from build123d import *

# Parameters (mm, degrees)
SKETCH1_W           = 36
SKETCH1_H           = 42
SKETCH1_R           = 1.55
BOSS_EXTRUDE1_DEPTH = 2
SKETCH5_W           = 42
SKETCH5_H           = 9.1
BOSS_EXTRUDE2_DEPTH = 7.4
SKETCH6_W           = 10
SKETCH6_H           = 9.1
BOSS_EXTRUDE3_DEPTH = 2
SKETCH2_R           = 3
CUT_EXTRUDE1_DEPTH  = 6
SKETCH4_W           = 16
SKETCH4_H           = 1.45
BOSS_EXTRUDE4_DEPTH = 0.4
FILLET2_R           = 3
FILLET3_R           = 0.5
SKETCH7_W           = 29
SKETCH7_H           = 20
BOSS_EXTRUDE5_DEPTH = 6
SKETCH8_W           = 20
SKETCH8_H           = 20
SKETCH8_R           = 8
SKETCH8_R_2         = 1.05
BOSS_EXTRUDE6_DEPTH = 3
FILLET4_R           = 2
SKETCH10_W          = 24
SKETCH10_H          = 19
SKETCH10_R          = 2.6
BOSS_EXTRUDE7_DEPTH = 3
SKETCH14_W          = 26
SKETCH14_H          = 25
BOSS_EXTRUDE8_DEPTH = 10.5
CUT_EXTRUDE3_REACH  = 60.08
SKETCH9_R           = 3.25
CUT_EXTRUDE2_DEPTH  = 13
FILLET6_R           = 1
FILLET7_R           = 1
FILLET8_R           = 4
FILLET9_R           = 1
FILLET10_R          = 1


with BuildPart() as part:
    # Sketch1 → Boss-Extrude1 (new body)
    with BuildSketch(Plane(origin=(0, 0, 0), x_dir=(0, 1, 0), z_dir=(0, 0, 1))):
        with Locations((5, 0)):
            Rectangle(SKETCH1_W, SKETCH1_H)
        with Locations(Location((-10, -10, 0), (0, 0, 270))):
            Circle(SKETCH1_R, mode=Mode.SUBTRACT)
        with Locations(Location((10, -10, 0), (0, 0, 270))):
            Circle(SKETCH1_R, mode=Mode.SUBTRACT)
        with Locations(Location((10, 10, 0), (0, 0, 270))):
            Circle(SKETCH1_R, mode=Mode.SUBTRACT)
        with Locations(Location((-10, 10, 0), (0, 0, 270))):
            Circle(SKETCH1_R, mode=Mode.SUBTRACT)
    extrude(amount=BOSS_EXTRUDE1_DEPTH)

    # Sketch5 → Boss-Extrude2 (add)
    with BuildSketch(Plane.XY):
        with Locations((0, 18.45)):
            Rectangle(SKETCH5_W, SKETCH5_H)
    extrude(amount=-BOSS_EXTRUDE2_DEPTH)

    # Sketch6 → Boss-Extrude3 (add)
    with BuildSketch(Plane(origin=(0, 0, -7.4), x_dir=(1, 0, 0), z_dir=(0, 0, -1))):
        with Locations((0, -18.45)):
            Rectangle(SKETCH6_W, SKETCH6_H)
    extrude(amount=BOSS_EXTRUDE3_DEPTH)

    # Sketch2 → Cut-Extrude1 (cut)
    with BuildSketch(Plane(origin=(0, 0, -9.4), x_dir=(1, 0, 0), z_dir=(0, 0, -1))):
        with Locations(Location((0, -18.5, 0), (0, 0, 180))):
            Circle(SKETCH2_R)
    extrude(amount=-CUT_EXTRUDE1_DEPTH, mode=Mode.SUBTRACT)

    # Sketch4 → Boss-Extrude4 (add)
    with BuildSketch(Plane(origin=(0, 0, -7.4), x_dir=(1, 0, 0), z_dir=(0, 0, -1))):
        with Locations((-13, -14.625)):
            Rectangle(SKETCH4_W, SKETCH4_H)
        with Locations((-13, -22.275)):
            Rectangle(SKETCH4_W, SKETCH4_H)
        with Locations((13, -14.625)):
            Rectangle(SKETCH4_W, SKETCH4_H)
        with Locations((13, -22.275)):
            Rectangle(SKETCH4_W, SKETCH4_H)
    extrude(amount=BOSS_EXTRUDE4_DEPTH)

    # Fillet2
    fillet2_edges = [part.edges().sort_by_distance(p)[0] for p in [
        (-21, -13, 1),
        (21, -13, 1),
    ]]
    fillet(fillet2_edges, radius=FILLET2_R)

    # Fillet3
    fillet3_edges = [part.edges().sort_by_distance(p)[0] for p in [
        (-5, 18.45, -9.4),
        (5, 18.45, -9.4),
    ]]
    fillet(fillet3_edges, radius=FILLET3_R)

    # Sketch7 → Boss-Extrude5 (add)
    with BuildSketch(Plane.XY.offset(2)):
        with Locations((-6.5, 0)):
            Rectangle(SKETCH7_W, SKETCH7_H)
    extrude(amount=BOSS_EXTRUDE5_DEPTH)

    # Sketch8 → Boss-Extrude6 (add)
    with BuildSketch(Plane(origin=(-21, 0, 0), x_dir=(0, -1, 0), z_dir=(-1, 0, 0))):
        with Locations((0, 18)):
            Rectangle(SKETCH8_W, SKETCH8_H)
        with Locations(Location((0, 18, 0), (0, 0, 90))):
            Circle(SKETCH8_R, mode=Mode.SUBTRACT)
        with Locations(Location((7.7, 25.7, 0), (0, 0, 90))):
            Circle(SKETCH8_R_2, mode=Mode.SUBTRACT)
        with Locations(Location((7.7, 10.3, 0), (0, 0, 90))):
            Circle(SKETCH8_R_2, mode=Mode.SUBTRACT)
        with Locations(Location((-7.7, 25.7, 0), (0, 0, 90))):
            Circle(SKETCH8_R_2, mode=Mode.SUBTRACT)
        with Locations(Location((-7.7, 10.3, 0), (0, 0, 90))):
            Circle(SKETCH8_R_2, mode=Mode.SUBTRACT)
    extrude(amount=-BOSS_EXTRUDE6_DEPTH)

    # Fillet4
    fillet4_edges = [part.edges().sort_by_distance(p)[0] for p in [
        (-19.5, 10, 28),
        (-19.5, -10, 28),
    ]]
    fillet(fillet4_edges, radius=FILLET4_R)



with BuildPart() as body_2:
    # Sketch10 → Boss-Extrude7 (new body)
    with BuildSketch(Plane(origin=(-10, 0, 0), x_dir=(0, 1, 0), z_dir=(-1, 0, 0))):
        with Locations((23, -22)):
            Rectangle(SKETCH10_W, SKETCH10_H)
        with Locations(Location((28.777800617, -22, 0), (0, 0, 270))):
            Circle(SKETCH10_R, mode=Mode.SUBTRACT)
        with Locations(Location((17.222199383, -22, 0), (0, 0, 270))):
            Circle(SKETCH10_R, mode=Mode.SUBTRACT)
    extrude(amount=BOSS_EXTRUDE7_DEPTH)


with BuildPart() as body_3:
    # Mirror1: mirrored copy
    add(body_2.part.mirror(Plane(origin=(0, 0, 0), x_dir=(0, 0, 1), z_dir=(1, 0, 0))))


with BuildPart() as part_1:
    add(part.part)

    add(body_2.part)  # Boss-Extrude8 merges body 2

    add(body_3.part)  # Boss-Extrude8 merges body 3
    # Sketch14 → Boss-Extrude8 (add)
    with BuildSketch(Plane(origin=(0, 0, 12.5), x_dir=(1, 0, 0), z_dir=(0, 0, -1))):
        with Locations((0, -22.5)):
            Rectangle(SKETCH14_W, SKETCH14_H)
    extrude(amount=BOSS_EXTRUDE8_DEPTH)

    # Cut-Extrude3: up to this face of the body (flat: up to its plane)
    cut_extrude3_end = Plane(part_1.part.faces().sort_by_distance((-13, 22.805850567, 16.272591727))[0])
    # Sketch15 → Cut-Extrude3 (cut, up to the picked face)
    with BuildSketch(Plane.YZ.offset(13), mode=Mode.PRIVATE) as cut_extrude3_sk1:
        with BuildLine():
            Line((23, 2), (29.749203665, 7.905553207))
            ThreePointArc((29.749203665, 7.905553207), (33.625901319, 13.123522322), (35, 19.477091335))
            Line((35, 19.477091335), (35, 12.5))
            Line((35, 12.5), (35, 2))
            Line((35, 2), (23, 2))
        make_face()
    cut_extrude3_tool1 = split(extrude(cut_extrude3_sk1.sketch, amount=-CUT_EXTRUDE3_REACH, mode=Mode.PRIVATE), bisect_by=cut_extrude3_end, keep=Keep.BOTH, mode=Mode.PRIVATE)
    # Sketch15 → Cut-Extrude3 (cut, up to the picked face)
    with BuildSketch(Plane.YZ.offset(13), mode=Mode.PRIVATE) as cut_extrude3_sk2:
        Polygon((12.370074724, 12.5), (10, 8), (10, 12.5), align=None)
    cut_extrude3_tool2 = split(extrude(cut_extrude3_sk2.sketch, amount=-CUT_EXTRUDE3_REACH, mode=Mode.PRIVATE), bisect_by=cut_extrude3_end, keep=Keep.BOTH, mode=Mode.PRIVATE)
    add(cut_extrude3_tool1.solids().sort_by(Axis((13, 31.275358, 6.207395), (-1, 0, 0)))[0], mode=Mode.SUBTRACT)
    add(cut_extrude3_tool2.solids().sort_by(Axis((13, 10.790025, 11), (-1, 0, 0)))[0], mode=Mode.SUBTRACT)

    # Sketch9 → Cut-Extrude2 (cut)
    with BuildSketch(Plane.XY.offset(2)):
        with Locations((-10, 10)):
            Circle(SKETCH9_R)
        with Locations((10, 10)):
            Circle(SKETCH9_R)
        with Locations((10, -10)):
            Circle(SKETCH9_R)
        with Locations((-10, -10)):
            Circle(SKETCH9_R)
    extrude(amount=CUT_EXTRUDE2_DEPTH, mode=Mode.SUBTRACT)

    # Fillet6
    # the kernel refuses this fillet: 1 mm, written as the material it takes off along each edge
    with BuildSketch(Plane(origin=(-13, 11.25, 15), x_dir=(0, 1, 0), z_dir=(0, 0, -1))) as fillet6_piece_1:
        with BuildLine():
            CenterArc((2.5, 1), FILLET6_R, 151.927513064, 118.072486936)
            ThreePointArc((1.617647059, 1.470588235), (0.93618658, 0.595194761), (0, 0))
            Line((0, 0), (2.5, 0))
        make_face()
    extrude(amount=8.75, mode=Mode.SUBTRACT)
    with BuildSketch(Plane(origin=(-13, 11.25, 16.623342892), x_dir=(0, 1, 0), z_dir=(0, 0, -1))) as fillet6_piece_2_section:
        with BuildLine():
            CenterArc((2.5, 1), FILLET6_R, 151.927513064, 118.072486936)
            ThreePointArc((1.617647059, 1.470588235), (0.93618658, 0.595194761), (0, 0))
            Line((0, 0), (2.5, 0))
        make_face()
    fillet6_piece_2 = extrude(amount=14.623342892, mode=Mode.PRIVATE)
    fillet6_piece_2 = split(fillet6_piece_2, bisect_by=Plane(origin=(-12.647638468, 12.372868888, 15), z_dir=(0, 0, -1)), keep=Keep.TOP, mode=Mode.PRIVATE)
    add(fillet6_piece_2, mode=Mode.SUBTRACT)
    with BuildSketch(Plane(origin=(-13.25, 10, 10.201694776), x_dir=(-1, 0, 0), z_dir=(0, 0, -1))) as fillet6_piece_3:
        with BuildLine():
            CenterArc((0.88067791, -1), FILLET6_R, 90, 76.391039369)
            ThreePointArc((-0.091246304, -0.764705882), (-0.022892199, -0.385065246), (0, 0))
            Line((0, 0), (0.88067791, 0))
        make_face()
    extrude(amount=8.201694776, mode=Mode.SUBTRACT)
    with BuildSketch(Plane(origin=(-6.75, -10, 2), x_dir=(1, 0, 0), z_dir=(0, 0, 1)), Plane(origin=(-13.25, -10, 10.201694776), x_dir=(-1, 0, 0), z_dir=(0, 0, -1))) as fillet6_piece_4:
        with BuildLine():
            CenterArc((0.88067791, 1), FILLET6_R, 193.608960631, 76.391039369)
            ThreePointArc((-0.091246304, 0.764705882), (-0.022892199, 0.385065246), (0, 0))
            Line((0, 0), (0.88067791, 0))
        make_face()
    extrude(amount=8.201694776, mode=Mode.SUBTRACT)
    with BuildSketch(Plane(origin=(8, -7.438262309, 9.121652383), x_dir=(0, 1, 0), z_dir=(0, 0, -1))) as fillet6_piece_5:
        with BuildLine():
            CenterArc((0.448660953, -1), FILLET6_R, 90, 45.099127844)
            ThreePointArc((-0.25966814, -0.294117647), (-0.125391755, -0.150980818), (0, 0))
            Line((0, 0), (0.448660953, 0))
        make_face()
    extrude(amount=7.121652383, mode=Mode.SUBTRACT)
    with BuildSketch(Plane(origin=(6.75, -10, 10.201694776), x_dir=(0.11848161412860787, 0.9929562463238145, 0), z_dir=(0, 0, -1))) as fillet6_piece_6:
        with BuildLine():
            CenterArc((0.888612106, -0.992956246), FILLET6_R, 96.804480315, 76.391039369)
            Line((-0.10434414, -0.874474632), (0, 0))
            ThreePointArc((0, 0), (0.385065246, -0.022892199), (0.770130492, 0))
        make_face()
    extrude(amount=8.201694776, mode=Mode.SUBTRACT)
    with BuildSketch(Plane(origin=(13, 11.25, 16.623342892), x_dir=(0, 1, 0), z_dir=(0, 0, -1))) as fillet6_piece_7_section:
        with BuildLine():
            CenterArc((2.5, -1), FILLET6_R, 90, 118.072486936)
            ThreePointArc((1.617647059, -1.470588235), (0.93618658, -0.595194761), (0, 0))
            Line((0, 0), (2.5, 0))
        make_face()
    fillet6_piece_7 = extrude(amount=14.623342892, mode=Mode.PRIVATE)
    fillet6_piece_7 = split(fillet6_piece_7, bisect_by=Plane(origin=(12.647638468, 12.372868888, 15), z_dir=(0, 0, -1)), keep=Keep.TOP, mode=Mode.PRIVATE)
    add(fillet6_piece_7, mode=Mode.SUBTRACT)
    with BuildSketch(Plane(origin=(13, 11.25, 15), x_dir=(0, 1, 0), z_dir=(0, 0, -1))) as fillet6_piece_8:
        with BuildLine():
            CenterArc((2.5, -1), FILLET6_R, 90, 118.072486936)
            ThreePointArc((1.617647059, -1.470588235), (0.93618658, -0.595194761), (0, 0))
            Line((0, 0), (2.5, 0))
        make_face()
    extrude(amount=8.75, mode=Mode.SUBTRACT)
    with BuildSketch(Plane(origin=(9.285048768, 12.370074724, 12.5), x_dir=(0, 1, 0), z_dir=(-1, 0, 0))) as fillet6_piece_9:
        with BuildLine():
            CenterArc((FILLET6_R * 0.603535852363, FILLET6_R), FILLET6_R, 207.775026011, 62.224973989)
            Line((-FILLET6_R * 0.281248326648, FILLET6_R * 0.533998973637), (0, 0))
            Line((0, 0), (FILLET6_R * 0.603535852363, 0))
        make_face()
    extrude(amount=18.570097535, mode=Mode.SUBTRACT)

    # Fillet7
    fillet7_edges = [part_1.edges().sort_by_distance(p)[0] for p in [
        (11.5, 11, 15),
        (-11.5, 11, 15),
    ]]
    fillet(fillet7_edges, radius=FILLET7_R)

    # Fillet8
    fillet8_edges = [part_1.edges().sort_by_distance(p)[0] for p in [
        (0, 23, 2),
        (-11.5, 35, 31.5),
        (-11.5, 11, 31.5),
        (11.5, 11, 31.5),
        (11.5, 35, 31.5),
    ]]
    fillet(fillet8_edges, radius=FILLET8_R)

    # Fillet9
    fillet9_edges = [part_1.edges().sort_by_distance(p)[0] for p in [
        (17, 23, 2),
        (-17, 23, 2),
    ]]
    fillet(fillet9_edges, radius=FILLET9_R)

    # Fillet10
    fillet10_edges = [part_1.edges().sort_by_distance(p)[0] for p in [
        (0, 33.325868907, 12.5),
    ]]
    fillet(fillet10_edges, radius=FILLET10_R)


solid = part_1.part
Geometry: final body of the model. Coordinates: model frame, mm. A direction names the side the tool comes from. Round coordinates to 2 decimals unless told otherwise and drop trailing zeros. Order: outer loops, then holes, each group sorted by start corner. A loop starts at its lowest first (then second) coordinate and runs counter-clockwise, first axis right, second up.
Q1. Access query for faces 1 (the face through (11.5, 12.5, 15)), 2 (the face through (-11, 11, 22)), 3 (the face through (-19, 10, 11)), 4 (the face through (-5, 0, 8)). Directions: +Z, -Z, +X, -X, +Y, -Y. A direction counts if a zero-diameter tool reaches every point of the face in a straight line with its end or side. Return the directions, or none.
Result sheet:
face 1: -Y
face 2: +Z, +X, -X, -Y
face 3: +Z, -X, +Y
face 4: +Z, +X, -Y
Q2. Section B-B, the plane z = 18. Output: boundary loops of the cut face in (x, y).
Result sheet:
outline: (-21, -10) - (-18, -10) - (-18, -8) - (-21, -8) - close; (-21, 8) - (-18, 8) - (-18, 10) - (-21, 10) - close; (-13, 11) - (-10, 11) - (-10, 34.93) - (-13, 34.93) - close; (10, 11) - (13, 11) - (13, 34.93) - (10, 34.93) - close
Q3. Pin query (flat end, axial travel): pin 1 (1 mm diameter, centred on x = 16.5, y = 13, fed in from -Z); pin 2 (1.2 mm diameter, centred on x = 11.5, y = 22, fed in from -Z); pin 3 (6 mm diameter, centred on x = -10, z = 0, fed in from +Y); pin 4 (12 mm diameter, centred on y = 12, z = 24.5, fed in from -X). Return the tip coordinate at first contact, or that it passes through.
Result sheet:
pin 1: stops at z = 0
pin 2: stops at z = -7.8
pin 3: stops at y = 24.16
pin 4: stops at x = -21
Q4. Section D-D, the plane x = 0. Output: boundary loops of the cut face in (y, z).
Result sheet:
outline: (-13, 0) - (13.9, 0) - (13.9, -9.4) - (15.5, -9.4) - (15.5, -3.4) - (21.5, -3.4) - (21.5, -9.4) - (23, -9.4) - (23, 0.18) arc R4 cw to (24.37, 3.2) - (29.75, 7.91) arc R15.38 ccw to (32.42, 10.95) arc R1 ccw to (31.58, 12.5) - (12.97, 12.5) arc R1 ccw to (12.09, 11.97) - (10, 8) - (-10, 8) - (-10, 2) - (-13, 2) - close
Q5. Section A-A, the plane x = 16.5. Output: boundary loops of the cut face in (y, z), and give its area (3 significant figures).
Result sheet:
outline: (-13, 0) - (13.9, 0) - (13.9, -7.8) - (15.35, -7.8) - (15.35, -7.4) - (21.55, -7.4) - (21.55, -7.8) - (23, -7.8) - (23, 1) arc R1 ccw to (22, 2) - (-13, 2) - close
area: 140 mm2
Q6. Mould query, pull axis X, two halves, no side actions, for faces 5 (the face through (13, 22, -7.8)), 6 (the face through (20.14, -12.1, 1.01)), 7 (the face through (-10, 23, 23)). Classes: released by +X, released by -X, zero draft, split by the parting line, or undercut.
Result sheet:
face 5: zero draft
face 6: released by +X
face 7: undercut
Q7. Section C-C, the plane y = -1.5. Output: boundary loops of the cut face in (x, z), and give its area (3 significant figures).
Result sheet:
outline: (-21, 0) - (21, 0) - (21, 2) - (8, 2) - (8, 8) - (-18, 8) - (-18, 10.14) - (-21, 10.14) - close; (-21, 25.86) - (-18, 25.86) - (-18, 28) - (-21, 28) - close
area: 271 mm2
Q8. Material intervals for probe 1 along X at (y, z) = (11.5, 19.5); probe 2 along Y at (x, z) = (-12.5, -5.5); probe 3 along Z at (x, y) = (19.5, 4.5), sorted ascending.
Result sheet:
probe 1: x = -13 to -10, 10 to 13
probe 2: y = 13.9 to 23
probe 3: z = 0 to 2
